Autodesk Fusion 360 part; units mm, degrees
sketch "Sketch1" plane through (0, 0, 0) normal (0, 1, 0) x (1, 0, 0)
  line L0 (-4.8, 0) -> (-4.8, -10)
  line L1 (0, 0) -> (0, -15)
  line L2 (0, -15) -> (-4.8, -15)
  line L3 (0, 0) -> (-4.8, 0) construction
  line L4 (-4.8, 0) -> (-4.8, 7.5)
  line L5 (0, -30) -> (-4.8, -30)
  line L6 (0, -15) -> (0, -30) construction
  line L7 (-4.8, -15) -> (-4.8, -30) construction
  line L8 (-4.8, -30) -> (-9.8, -30)
  line L9 (-14.8, 7.5) -> (-14.8, -25)
  arc A0 (-9.8, -30) -> (-14.8, -25) centre (-9.8, -25) ccw construction
  arc A1 (-14.8, -25) -> (-9.8, -30) centre (-9.8, -25) ccw
  arc A2 (-14.8, 7.5) -> (-4.8, 7.5) centre (-9.8, 7.5) ccw construction
  arc A3 (-4.8, 7.5) -> (-14.8, 7.5) centre (-9.8, 7.5) ccw
  circle A4 centre (-9.8, 7.5) radius 1.5
  line L10 (0, 0) -> (5, 0)
  line L11 (5, 0) -> (5, -4.8)
  line L12 (5, -4.8) -> (15, -4.8)
  line L13 (15, -4.8) -> (15, 0)
  line L14 (15, 0) -> (20, 0)
  line L15 (20, 0) -> (20, 7.5)
  line L16 (30, 7.5) -> (30, -5)
  line L17 (3.1235, -28.9043) -> (28.1235, -8.9043)
  arc A5 (3.1235, -28.9043) -> (0, -30) centre (0, -25) ccw construction
  arc A6 (0, -30) -> (3.1235, -28.9043) centre (0, -25) ccw
  arc A7 (30, -5) -> (28.1235, -8.9043) centre (25, -5) ccw construction
  arc A8 (28.1235, -8.9043) -> (30, -5) centre (25, -5) ccw
  arc A9 (20, 7.5) -> (30, 7.5) centre (25, 7.5) ccw construction
  arc A10 (30, 7.5) -> (20, 7.5) centre (25, 7.5) ccw
  circle A11 centre (25, 7.5) radius 1.5
  line L18 (-4.8, -10) -> (-9.6, -10)
  line L19 (-9.6, -10) -> (-9.6, -20)
  line L20 (-9.6, -20) -> (-4.8, -20)
  line L21 (-4.8, -20) -> (-4.8, -15)
  line L22 (-9.8, 7.5) -> (-9.8, -25) construction
  line L23 (-4.8, 7.5) -> (20, 7.5) construction
  dimension "d1" = 15
  dimension "d3" = 4.8
  dimension "d4" = 7.5
  dimension "d5" = 4.8
  dimension "d6" = 15
  dimension "d7" = 10
  dimension "d8" = 10
  dimension "d9" = 3
  dimension "d10" = 5
  dimension "d11" = 4.8
  dimension "d12" = 10
  dimension "d13" = 4.8
  dimension "d14" = 5
  dimension "d16" = 10
  dimension "d17" = 10
  dimension "d18" = 5
  dimension "d19" = 5
  dimension "d20" = 5
  dimension "d21" = 3
  dimension "d22" = 4.8
  dimension "d23" = 10
  dimension "d24" = 5
extrude "Extrude1" add sketch "Sketch1" along normal blind 4.8
Part model, mm, in its own coordinate system. A direction names the side the tool comes from. Give positions to 0.01 mm unless a question says otherwise; leave off trailing zeros. Write each loop counter-clockwise with the first axis right and the second up, starting at its lowest first coordinate (ties: lowest second). Pieces come first, ordered by that corner, then holes. Notation, with made-up numbers: M 2.25,44.5 L 54.25,44.5 A22 cw 54.25,65.5 Z; hole C -9.75,11.25 d11. An arc over 180 degrees is marked long. Use CSV: the item, a comma, the result in double quotes.
Item 1: Slice it at D-D on z = -8. Write the cut outline in (x, y).
Taken from the geometry:
outline,"M -14.77,0 L -11.21,0 L -11.21,4.8 L -14.77,4.8 Z; M -8.39,0 L -4.83,0 L -4.83,4.8 L -8.39,4.8 Z; M 20.03,0 L 23.59,0 L 23.59,4.8 L 20.03,4.8 Z; M 26.41,0 L 29.97,0 L 29.97,4.8 L 26.41,4.8 Z"
Item 2: Slice it at C-C on x = -6. Write the cut outline in (y, z), plus the area to 3 significant figures.
Taken from the geometry:
outline,"M 0,-10.75 L 4.8,-10.75 L 4.8,10 L 0,10 Z; M 0,20 L 4.8,20 L 4.8,30 L 0,30 Z"
area,"148 mm²"
Item 3: Slice it at B-B on y = 2.8. Write the cut outline in (x, z).
Taken from the geometry:
outline,"M -14.8,-7.5 A5 ccw -4.8,-7.5 L -4.8,10 L -9.6,10 L -9.6,20 L -4.8,20 L -4.8,15 L 0,15 L 0,0 L 5,0 L 5,4.8 L 15,4.8 L 15,0 L 20,0 L 20,-7.5 A5 ccw 30,-7.5 L 30,5 A5 ccw 28.12,8.9 L 3.12,28.9 A5 ccw 0,30 L -9.8,30 A5 ccw -14.8,25 Z; hole C -9.8,-7.5 d3; hole C 25,-7.5 d3"
Item 4: Pin check, flat tips, straight feed: P1, Ø2.5, axis at x = -6, y = 2, coming from the -Z side; P2, Ø1.4, axis at y = 3, z = 17, coming from the +X side; P3, Ø1.5, axis at x = 8.5, y = 2, coming from the +Z side. Stop position of each tip, or through.
Taken from the geometry:
P1,"stops at z = -11.8"
P2,"stops at x = 18.88"
P3,"stops at z = 25.2"
Item 5: Which spindle directions (+Z, -Z, +X, -X, +Y, -Y) get a long thin tool onto all of the face, cutting with end or side? Do faces 5 (the face through (-14.8, 2, 9)), 6 (the face through (-4.8, 2, 18)), 7 (the face through (0, 2, 7)). Say none if no direction does.
Taken from the geometry:
face 5,"+Z, -Z, -X, +Y, -Y"
face 6,"+Y, -Y"
face 7,"-Z, +Y, -Y"
Item 6: Pull direction X, two halves, no side cores. Call faces 1 (the face through (30, 2, -1)), 2 (the face through (7, 4.8, 8)), 3 (the face through (17, 2, 0)), 4 (the face through (-9.6, 2, 15)): +X half, -X half, draft (parallel to the pull), parting line (faces both ways), or undercut.
Taken from the geometry:
face 1,"+X half"
face 2,"draft"
face 3,"undercut"
face 4,"undercut"
Item 7: Drill centre lines: probe 1 along X at (y, z) = (3.1, -7.5); probe 2 along X at (y, z) = (3.75, 2); probe 3 along Z at (x, y) = (-9.8, 2.75). Where is each one in solid material? Low to high.
Taken from the geometry:
probe 1,"x = -14.8 to -11.3, -8.3 to -4.8, 20 to 23.5, 26.5 to 30"
probe 2,"x = -14.8 to -4.8, 0 to 5, 15 to 30"
probe 3,"z = -12.5 to -9, -6 to 30"
Item 8: Slice it at A-A on z = -1. Write the cut outline in (x, y), plus the area to 3 significant figures.
Taken from the geometry:
outline,"M -14.8,0 L -4.8,0 L -4.8,4.8 L -14.8,4.8 Z; M 20,0 L 30,0 L 30,4.8 L 20,4.8 Z"
area,"96.0 mm²"
